Source: CAD feature listing. Evaluate the final solid. Frame: model axes, mm. Face numbers are marked on the shaded views. A direction names the side the tool comes from. Give positions to 0.01 mm unless a question says otherwise; leave off trailing zeros. Write each loop counter-clockwise with the first axis right and the second up, starting at its lowest first coordinate (ties: lowest second). Pieces come first, ordered by that corner, then holes. Notation, with made-up numbers: (-28, 84) -> (9, 84) arc R25 cw to (9, 108) -> close; hole circle Ø7 at (23.5, 83). An arc over 180 degrees is marked (long way). Answer as a JSON object with one key per item and string values. Group by question number.
Item 1: Section query B-B on y = 0. Return the cut outline in (x, z).
Item 2: Section query C-C on z = -1. Return the cut outline in (x, y).
Item 3: Section query D-D on x = -5. Return the cut outline in (y, z) (3 decimals).
Item 4: Section query A-A on x = 0. Return the cut outline in (y, z), plus the area to 3 significant figures.
Item 5: Access query for the marked faces 1 and 2. Directions: +Z, -Z, +X, -X, +Y, -Y. A direction counts if a zero-diameter tool reaches every point of the face in a straight line with its end or side. Return the directions, or none.
Item 6: Ray query, probe 1 along Z at (x, y) = (2.25, 6.5); probe 2 along X at (y, z) = (-0.25, -9); probe 3 along X at (y, z) = (1.5, 6.5). Return the intervals inside material, ascending. Write a range as from..to.
Item 7: First-contact query: pin 1 Ø5 at (x, y) = (0.5, 3) entering from +Z; pin 2 Ø2.5 at (y, z) = (-0.5, 3.5) entering from +X; pin 3 Ø2.5 at (y, z) = (0, 3) entering from -X; pin 4 Ø6 at (x, z) = (-2, -10.5) entering from -Y. Flat tips, straight axial feed; report the tip coordinate or a pass-through.
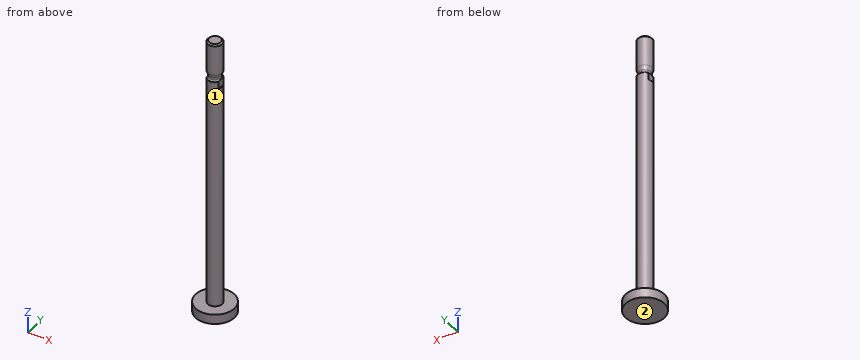
from build123d import *

# Parameters (mm, degrees)
CUT_EXTRUDE1_DEPTH = 4


with BuildPart() as part:
    # Sketch1 → Revolve1 (revolve)
    with BuildSketch(Plane(origin=(0, 0, 0), x_dir=(0, 0, -1), z_dir=(1, 0, 0))):
        Polygon((-5, 0), (-5, 3), (91.2, 3), (91.2, 8), (95.2, 8), (95.2, 0), align=None)
    revolve(axis=Axis((0, 0, -95.2), (0, 0, 1)))

    # Sketch2 → Revolve2 (revolve)
    with BuildSketch(Plane(origin=(0, 0, 0), x_dir=(0, 0, -1), z_dir=(1, 0, 0))):
        with BuildLine():
            Line((-21, 0), (-21, 2.3865))
            Line((-21, 2.3865), (-20.3865, 3))
            Line((-20.3865, 3), (-8.148486452, 3))
            Line((-8.148486452, 3), (-6.599415898, 2.436184428))
            ThreePointArc((-6.599415898, 2.436184428), (-6.498392718, 2.409115348), (-6.394203812, 2.4))
            Line((-6.394203812, 2.4), (-5.6, 2.4))
            ThreePointArc((-5.6, 2.4), (-5.175735931, 2.575735931), (-5, 3))
            Line((-5, 3), (-4, 3))
            Line((-4, 3), (-4, 0))
            Line((-4, 0), (-21, 0))
        make_face()
    revolve(axis=Axis((0, 0, 4), (0, 0, 1)))

    # Sketch3 → Cut-Extrude1 (cut)
    with BuildSketch(Plane.XY.offset(2)):
        Polygon((-5, 10), (-5, -5), (-2.5, -5), (-2.5, 5), (2.5, 5), (2.5, -5), (5, -5), (5, 10), align=None)
    extrude(amount=CUT_EXTRUDE1_DEPTH, mode=Mode.SUBTRACT)


solid = part.part
Worked answers:
{
 "1": {"outline": "(-8, -95.2) -> (8, -95.2) -> (8, -91.2) -> (3, -91.2) -> (3, 2) -> (2.5, 2) -> (2.5, 5.27) arc R0.6 cw to (2.4, 5.6) -> (2.4, 6.39) arc R0.6 cw to (2.44, 6.6) -> (3, 8.15) -> (3, 20.39) -> (2.39, 21) -> (-2.39, 21) -> (-3, 20.39) -> (-3, 8.15) -> (-2.44, 6.6) arc R0.6 cw to (-2.4, 6.39) -> (-2.4, 5.6) arc R0.6 cw to (-2.5, 5.27) -> (-2.5, 2) -> (-3, 2) -> (-3, -91.2) -> (-8, -91.2) -> close"},
 "2": {"outline": "circle Ø6 at (0, 0)"},
 "3": {"outline": "(-6.245, -95.2) -> (6.245, -95.2) -> (6.245, -91.2) -> (-6.245, -91.2) -> close"},
 "4": {"outline": "(-8, -95.2) -> (8, -95.2) -> (8, -91.2) -> (3, -91.2) -> (3, 5) arc R0.6 cw to (2.4, 5.6) -> (2.4, 6.39) arc R0.6 cw to (2.44, 6.6) -> (3, 8.15) -> (3, 20.39) -> (2.39, 21) -> (-2.39, 21) -> (-3, 20.39) -> (-3, 8.15) -> (-2.44, 6.6) arc R0.6 cw to (-2.4, 6.39) -> (-2.4, 5.6) arc R0.6 cw to (-3, 5) -> (-3, -91.2) -> (-8, -91.2) -> close", "area": "734 mm^2"},
 "5": {"face 1": "+Z", "face 2": "-Z, +X, -X, +Y, -Y"},
 "6": {"probe 1": "-95.2..-91.2", "probe 2": "-2.99..2.99", "probe 3": "-1.89..1.89"},
 "7": {"pin 1": "z = 21", "pin 2": "x = 2.5", "pin 3": "x = -3", "pin 4": "y = -3"}
}
